```python
from build123d import *

# Parameters (mm, degrees)
SKETCH_1_R      = 2.5
EXTRUDE_1_DEPTH = 10


with BuildPart() as part:
    # 草图1 → 凸台-拉伸1 (new, symmetric)
    with BuildSketch(Plane.XY):
        with BuildLine():
            Line((10, 8.5), (10, 4))
            ThreePointArc((10, 4), (9.912132034, 3.787867966), (9.7, 3.7))
            ThreePointArc((9.7, 3.7), (9.487867966, 3.612132034), (9.4, 3.4))
            ThreePointArc((9.4, 3.4), (9.312132034, 3.187867966), (9.1, 3.1))
            Line((9.1, 3.1), (8.5, 3.1))
            ThreePointArc((8.5, 3.1), (8.287867966, 3.187867966), (8.2, 3.4))
            Line((8.2, 3.4), (8.2, 5.2))
            ThreePointArc((8.2, 5.2), (8.112132034, 5.412132034), (7.9, 5.5))
            Line((7.9, 5.5), (6.68492424, 5.5))
            ThreePointArc((6.68492424, 5.5), (6.570119211, 5.47716386), (6.472792206, 5.412132034))
            Line((6.472792206, 5.412132034), (4.485786438, 3.425126266))
            ThreePointArc((4.485786438, 3.425126266), (4.052240935, 2.776279568), (3.9, 2.010912703))
            Line((3.9, 2.010912703), (3.9, -2.010912703))
            ThreePointArc((3.9, -2.010912703), (4.052240935, -2.776279568), (4.485786438, -3.425126266))
            Line((4.485786438, -3.425126266), (6.472792206, -5.412132034))
            ThreePointArc((6.472792206, -5.412132034), (6.570119211, -5.47716386), (6.68492424, -5.5))
            Line((6.68492424, -5.5), (7.9, -5.5))
            ThreePointArc((7.9, -5.5), (8.112132034, -5.412132034), (8.2, -5.2))
            Line((8.2, -5.2), (8.2, -3.4))
            ThreePointArc((8.2, -3.4), (8.287867966, -3.187867966), (8.5, -3.1))
            Line((8.5, -3.1), (9.1, -3.1))
            ThreePointArc((9.1, -3.1), (9.312132034, -3.187867966), (9.4, -3.4))
            ThreePointArc((9.4, -3.4), (9.487867966, -3.612132034), (9.7, -3.7))
            ThreePointArc((9.7, -3.7), (9.912132034, -3.787867966), (10, -4))
            Line((10, -4), (10, -8.5))
            ThreePointArc((10, -8.5), (9.560660172, -9.560660172), (8.5, -10))
            Line((8.5, -10), (4, -10))
            ThreePointArc((4, -10), (3.787867966, -9.912132034), (3.7, -9.7))
            ThreePointArc((3.7, -9.7), (3.612132034, -9.487867966), (3.4, -9.4))
            ThreePointArc((3.4, -9.4), (3.187867966, -9.312132034), (3.1, -9.1))
            Line((3.1, -9.1), (3.1, -8.5))
            ThreePointArc((3.1, -8.5), (3.187867966, -8.287867966), (3.4, -8.2))
            Line((3.4, -8.2), (5.2, -8.2))
            ThreePointArc((5.2, -8.2), (5.412132034, -8.112132034), (5.5, -7.9))
            Line((5.5, -7.9), (5.5, -6.68492424))
            ThreePointArc((5.5, -6.68492424), (5.47716386, -6.570119211), (5.412132034, -6.472792206))
            Line((5.412132034, -6.472792206), (3.425126266, -4.485786438))
            ThreePointArc((3.425126266, -4.485786438), (2.776279568, -4.052240935), (2.010912703, -3.9))
            Line((2.010912703, -3.9), (-2.010912703, -3.9))
            ThreePointArc((-2.010912703, -3.9), (-2.776279568, -4.052240935), (-3.425126266, -4.485786438))
            Line((-3.425126266, -4.485786438), (-5.412132034, -6.472792206))
            ThreePointArc((-5.412132034, -6.472792206), (-5.47716386, -6.570119211), (-5.5, -6.68492424))
            Line((-5.5, -6.68492424), (-5.5, -7.9))
            ThreePointArc((-5.5, -7.9), (-5.412132034, -8.112132034), (-5.2, -8.2))
            Line((-5.2, -8.2), (-3.4, -8.2))
            ThreePointArc((-3.4, -8.2), (-3.187867966, -8.287867966), (-3.1, -8.5))
            Line((-3.1, -8.5), (-3.1, -9.1))
            ThreePointArc((-3.1, -9.1), (-3.187867966, -9.312132034), (-3.4, -9.4))
            ThreePointArc((-3.4, -9.4), (-3.612132034, -9.487867966), (-3.7, -9.7))
            ThreePointArc((-3.7, -9.7), (-3.787867966, -9.912132034), (-4, -10))
            Line((-4, -10), (-8.5, -10))
            ThreePointArc((-8.5, -10), (-9.560660172, -9.560660172), (-10, -8.5))
            Line((-10, -8.5), (-10, -4))
            ThreePointArc((-10, -4), (-9.912132034, -3.787867966), (-9.7, -3.7))
            ThreePointArc((-9.7, -3.7), (-9.487867966, -3.612132034), (-9.4, -3.4))
            ThreePointArc((-9.4, -3.4), (-9.312132034, -3.187867966), (-9.1, -3.1))
            Line((-9.1, -3.1), (-8.5, -3.1))
            ThreePointArc((-8.5, -3.1), (-8.287867966, -3.187867966), (-8.2, -3.4))
            Line((-8.2, -3.4), (-8.2, -5.2))
            ThreePointArc((-8.2, -5.2), (-8.112132034, -5.412132034), (-7.9, -5.5))
            Line((-7.9, -5.5), (-6.68492424, -5.5))
            ThreePointArc((-6.68492424, -5.5), (-6.570119211, -5.47716386), (-6.472792206, -5.412132034))
            Line((-6.472792206, -5.412132034), (-4.485786438, -3.425126266))
            ThreePointArc((-4.485786438, -3.425126266), (-4.052240935, -2.776279568), (-3.9, -2.010912703))
            Line((-3.9, -2.010912703), (-3.9, 2.010912703))
            ThreePointArc((-3.9, 2.010912703), (-4.052240935, 2.776279568), (-4.485786438, 3.425126266))
            Line((-4.485786438, 3.425126266), (-6.472792206, 5.412132034))
            ThreePointArc((-6.472792206, 5.412132034), (-6.570119211, 5.47716386), (-6.68492424, 5.5))
            Line((-6.68492424, 5.5), (-7.9, 5.5))
            ThreePointArc((-7.9, 5.5), (-8.112132034, 5.412132034), (-8.2, 5.2))
            Line((-8.2, 5.2), (-8.2, 3.4))
            ThreePointArc((-8.2, 3.4), (-8.287867966, 3.187867966), (-8.5, 3.1))
            Line((-8.5, 3.1), (-9.1, 3.1))
            ThreePointArc((-9.1, 3.1), (-9.312132034, 3.187867966), (-9.4, 3.4))
            ThreePointArc((-9.4, 3.4), (-9.487867966, 3.612132034), (-9.7, 3.7))
            ThreePointArc((-9.7, 3.7), (-9.912132034, 3.787867966), (-10, 4))
            Line((-10, 4), (-10, 8.5))
            ThreePointArc((-10, 8.5), (-9.560660172, 9.560660172), (-8.5, 10))
            Line((-8.5, 10), (-4, 10))
            ThreePointArc((-4, 10), (-3.787867966, 9.912132034), (-3.7, 9.7))
            ThreePointArc((-3.7, 9.7), (-3.612132034, 9.487867966), (-3.4, 9.4))
            ThreePointArc((-3.4, 9.4), (-3.187867966, 9.312132034), (-3.1, 9.1))
            Line((-3.1, 9.1), (-3.1, 8.5))
            ThreePointArc((-3.1, 8.5), (-3.187867966, 8.287867966), (-3.4, 8.2))
            Line((-3.4, 8.2), (-5.2, 8.2))
            ThreePointArc((-5.2, 8.2), (-5.412132034, 8.112132034), (-5.5, 7.9))
            Line((-5.5, 7.9), (-5.5, 6.68492424))
            ThreePointArc((-5.5, 6.68492424), (-5.47716386, 6.570119211), (-5.412132034, 6.472792206))
            Line((-5.412132034, 6.472792206), (-3.425126266, 4.485786438))
            ThreePointArc((-3.425126266, 4.485786438), (-2.776279568, 4.052240935), (-2.010912703, 3.9))
            Line((-2.010912703, 3.9), (2.010912703, 3.9))
            ThreePointArc((2.010912703, 3.9), (2.776279568, 4.052240935), (3.425126266, 4.485786438))
            Line((3.425126266, 4.485786438), (5.412132034, 6.472792206))
            ThreePointArc((5.412132034, 6.472792206), (5.47716386, 6.570119211), (5.5, 6.68492424))
            Line((5.5, 6.68492424), (5.5, 7.9))
            ThreePointArc((5.5, 7.9), (5.412132034, 8.112132034), (5.2, 8.2))
            Line((5.2, 8.2), (3.4, 8.2))
            ThreePointArc((3.4, 8.2), (3.187867966, 8.287867966), (3.1, 8.5))
            Line((3.1, 8.5), (3.1, 9.1))
            ThreePointArc((3.1, 9.1), (3.187867966, 9.312132034), (3.4, 9.4))
            ThreePointArc((3.4, 9.4), (3.612132034, 9.487867966), (3.7, 9.7))
            ThreePointArc((3.7, 9.7), (3.787867966, 9.912132034), (4, 10))
            Line((4, 10), (8.5, 10))
            ThreePointArc((8.5, 10), (9.560660172, 9.560660172), (10, 8.5))
        make_face()
        Circle(SKETCH_1_R, mode=Mode.SUBTRACT)
    extrude(amount=EXTRUDE_1_DEPTH, both=True)


solid = part.part
```
Part model, mm, in its own coordinate system. A direction names the side the tool comes from. Give positions to 0.01 mm unless a question says otherwise; leave off trailing zeros. Loops run counter-clockwise (first coordinate to the right, second up) from the corner with the lowest first, then second, coordinate; pieces in that order, holes last. Notation, with made-up numbers: M -21.75,39.5 L 12.25,39.5 A21 cw 12.25,72.5 Z; hole C 84.5,-16 d5. An arc over 180 degrees is marked long. Return JSON: item names as keys, results as strings.
1) Drill centre lines: line 1 (X direction, y = -7.75, z = -4); line 2 (Y direction, x = 0, z = 0.25); line 3 (Y direction, x = 4.5, z = 0.25). Where is each one in solid material? Low to high.
Calculated:
{"line 1": "x = -10 to -5.5, 5.5 to 10", "line 2": "y = -3.9 to -2.5, 2.5 to 3.9", "line 3": "y = -10 to -8.2, -5.56 to -3.44, 3.44 to 5.56, 8.2 to 10"}
2) Pull direction X, two halves, no side cores. Call faces 4 (the face through (-6, -10, 0)), 5 (the face through (-5.5, -7, 0)), 6 (the face through (9.55, 9.57, 0.14)): released by +X, released by -X, zero draft, split by the parting line, or undercut.
Calculated:
{"face 4": "zero draft", "face 5": "undercut", "face 6": "released by +X"}
3) Flat gauge pins, fed straight in: pin 1 Ø1.2 at (y, z) = (1, -2.5) entering from +X; pin 2 Ø3 at (x, z) = (0, 0) entering from -Y; pin 3 Ø0.7 at (x, z) = (-9, -4.5) entering from +Y; pin 4 Ø4 at (x, y) = (5, -1.5) entering from +Z. Where does each tip first touch, or does it go through?
Calculated:
{"pin 1": "stops at x = 3.9", "pin 2": "stops at y = -3.9", "pin 3": "stops at y = 9.99", "pin 4": "stops at z = 10"}
4) 3-axis set-ups, long thin cutter, end or side, ignore diameter. For faces 1 (the face through (4.06, 2.79, 0.14)), 2 (the face through (6, -10, 0)), 3 (the face through (0, -3.9, 0)): which of +Z, -Z, +X, -X, +Y, -Y reach the whole face in a straight line?
Calculated:
{"face 1": "+Z, -Z", "face 2": "+Z, -Z, +X, -X, -Y", "face 3": "+Z, -Z, -Y"}
5) Saw through at A-A, the plane y = 0. List the corners of the cut face in (x, z), then the cut area to 3 significant figures.
Calculated:
{"outline": "M -3.9,-10 L -2.5,-10 L -2.5,10 L -3.9,10 Z; M 2.5,-10 L 3.9,-10 L 3.9,10 L 2.5,10 Z", "area": "56.0 mm2"}
